from build123d import *

# Parameters (mm, degrees)
SKETCH1_W           = 38
SKETCH1_H           = 10
BOSS_EXTRUDE1_DEPTH = 5
SKETCH3_W           = 5
SKETCH3_H           = 2
BOSS_EXTRUDE2_DEPTH = 4
CHAMFER1_SIZE       = 0.5
CHAMFER2_SIZE       = 0.5


with BuildPart() as part:
    # Sketch1 → Boss-Extrude1 (new body)
    with BuildSketch(Plane(origin=(0, 0, 0), x_dir=(1, 0, 0), z_dir=(0, 1, 0))):
        with Locations((19, 5)):
            Rectangle(SKETCH1_W, SKETCH1_H)
    extrude(amount=BOSS_EXTRUDE1_DEPTH)

    # Sketch2 → Cut-Revolve1 (revolve, cut)
    with BuildSketch(Plane(origin=(0, 5, 0), x_dir=(1, 0, 0), z_dir=(0, 1, 0))):
        Polygon((0, 5), (38, 5), (38, 4.5), (26.25, 4.5), (26.25, 3.6), (11.75, 3.6), (11.75, 4.5), (0, 4.5), align=None)
    revolve(axis=Axis((0, 5, -5), (1, 0, 0)), mode=Mode.SUBTRACT)

    # Sketch3 → Boss-Extrude2 (add)
    with BuildSketch(Plane(origin=(0, 5, 0), x_dir=(1, 0, 0), z_dir=(0, 1, 0))):
        with Locations((5.5, 7.5)):
            Rectangle(SKETCH3_W, SKETCH3_H)
        with Locations((32.5, 7.5)):
            Rectangle(SKETCH3_W, SKETCH3_H)
        with Locations((32.5, 2.500985925)):
            Rectangle(SKETCH3_W, SKETCH3_H)
        with Locations((5.5, 2.500985925)):
            Rectangle(SKETCH3_W, SKETCH3_H)
    extrude(amount=BOSS_EXTRUDE2_DEPTH)

    # Chamfer1
    chamfer1_edges = [part.edges().sort_by_distance(p)[0] for p in [
        (3, 5, -7.5),
        (8, 5, -7.5),
        (5.5, 5, -8.5),
        (30, 5, -7.5),
        (35, 5, -7.5),
        (32.5, 5, -8.5),
        (30, 5, -2.500985925),
        (32.5, 5, -1.500985925),
        (35, 5, -2.500985925),
        (3, 5, -2.500985925),
        (5.5, 5, -1.500985925),
        (8, 5, -2.500985925),
    ]]
    chamfer(chamfer1_edges, length=CHAMFER1_SIZE)

    # Chamfer2
    chamfer2_edges = [part.edges().sort_by_distance(p)[0] for p in [
        (3, 9, -7.5),
        (5.5, 9, -6.5),
        (8, 9, -7.5),
        (5.5, 9, -8.5),
        (30, 9, -7.5),
        (32.5, 9, -6.5),
        (35, 9, -7.5),
        (32.5, 9, -8.5),
        (30, 9, -2.500985925),
        (32.5, 9, -1.500985925),
        (35, 9, -2.500985925),
        (32.5, 9, -3.500985925),
        (3, 9, -2.500985925),
        (5.5, 9, -1.500985925),
        (8, 9, -2.500985925),
        (5.5, 9, -3.500985925),
    ]]
    chamfer(chamfer2_edges, length=CHAMFER2_SIZE)


solid = part.part
For this review, take the finished solid that the model builds, in its own axes (mm). A direction names the side the tool comes from. Coordinates: 2 decimals unless noted, no trailing zeros. Order: outer loops, then holes, each group sorted by start corner. A loop starts at its lowest first (then second) coordinate and runs counter-clockwise, first axis right, second up. Notation, with made-up numbers: (-32.5, -17.75) -> (25.5, -17.75) arc R32 cw to (25.5, 19.25) -> close; hole circle Ø7 at (85, 68.5). An arc over 180 degrees is marked (long way). Return JSON: item names as keys, results as strings.
1. We need section D-D on x = 21. Write out the cut boundary in (y, z), and give its area (3 significant figures).
Answer block:
{"outline": "(0, -10) -> (5, -10) -> (5, -6.4) arc R1.4 cw to (5, -3.6) -> (5, 0) -> (0, 0) -> close", "area": "46.9 mm²"}
2. We need section A-A on z = -5. Write out the cut boundary in (x, y).
Answer block:
{"outline": "(0, 0) -> (38, 0) -> (38, 4.5) -> (26.25, 4.5) -> (26.25, 3.6) -> (11.75, 3.6) -> (11.75, 4.5) -> (0, 4.5) -> close"}
3. Machinability: for faces 1 (the flat face through (8, 7, -2)), 2 (the flat face through (32, 7, -3.501)), 3 (the flat face through (35, 7, -7)), which of the approach directions +Z, -Z, +X, -X, +Y, -Y give a long, thin tool a straight path to every point of the face, cutting with its end or side? Answer none if there is none.
Answer block:
{"face 1": "+Z, -Z, +Y", "face 2": "+X, -X, +Y", "face 3": "+Z, -Z, +X, +Y"}
4. For line 1 (X direction, y = 6.25, z = -7); line 2 (Z direction, x = 6, y = 6); line 3 (Y direction, x = 13, z = -8.25), list the stretches that pass through material, from the lowest coordinate up. Write a range as from..to.
Answer block:
{"line 1": "3..8, 30..35", "line 2": "-8.5..-6.5, -3.5..-1.5", "line 3": "0..5"}
5. The part is to be moulded in two halves that separate along Z. For faces 4 (the flat face through (3, 7, -7)), 5 (the flat face through (19, 2, -10)), 6 (the cylindrical face through (18.9, 3.6, -5)), 7 (the flat face through (5, 7, -3.501)), say which applies: +Z half, -Z half, draft (parallel to the pull), parting line (faces both ways), or undercut.
Answer block:
{"face 4": "draft", "face 5": "-Z half", "face 6": "undercut", "face 7": "undercut"}
6. For pin 1 Ø1.5 at (x, y) = (4.5, 7.5) entering from +Z; pin 2 Ø1.6 at (y, z) = (6.5, -2.5) entering from -X; pin 3 Ø0.6 at (y, z) = (7, -7.5) entering from +X; pin 4 Ø5 at (y, z) = (1.5, -9) entering from -X, all flat-tipped, find the tip position at first contact; note any pin that passes through.
Answer block:
{"pin 1": "z = -1.5", "pin 2": "x = 3", "pin 3": "x = 35", "pin 4": "x = 0"}
7. We need section B-B on x = 9. Write out the cut boundary in (y, z), and give its area (3 significant figures).
Answer block:
{"outline": "(0, -10) -> (5, -10) -> (5, -5.5) arc R0.5 cw to (5, -4.5) -> (5, 0) -> (0, 0) -> close", "area": "49.6 mm²"}
8. We need section C-C on z = -2.5. Write out the cut boundary in (x, y), and give its area (3 significant figures).
Answer block:
{"outline": "(0, 0) -> (38, 0) -> (38, 5) -> (35.5, 5) -> (35, 5.5) -> (35, 8.5) -> (34.5, 9) -> (30.5, 9) -> (30, 8.5) -> (30, 5.5) -> (29.5, 5) -> (8.5, 5) -> (8, 5.5) -> (8, 8.5) -> (7.5, 9) -> (3.5, 9) -> (3, 8.5) -> (3, 5.5) -> (2.5, 5) -> (0, 5) -> close", "area": "230 mm²"}
